The figure shows three views and two pictorial views of one solid part (mm, origin at its lowest corner). Answer the questions. A direction names the side the tool comes from. Round coordinates to 2 decimals unless told otherwise and drop trailing zeros. Loops run counter-clockwise (first coordinate to the right, second up) from the corner with the lowest first, then second, coordinate; pieces in that order, holes last. Notation, with made-up numbers: (-2, 54) -> (43, 54) arc R22 ccw to (43, 64) -> close; hole circle Ø2 at (22, 24.5). An arc over 180 degrees is marked (long way). Use a Markdown table: item, result. Add a question column.
Q1. For a pull along Y with two mould halves and no side action, classify the marked faces 3, 4 and 5 as released by +Y, released by -Y, zero draft, split by the parting line, or undercut.
Q2. Which of the six approach directions +Z, -Z, +X, -X, +Y, -Y give full straight-line access (tool end or side, diameter ignored) to the marked faces 1 and 2?
Q3. Section D-D on z = 14 is taken. Give the vertices of the cut face in (x, y).
Q4. Section C-C on z = 8 is taken. Give the vertices of the cut face in (x, y), then the cut area to 3 significant figures.
Q5. Section A-A on y = 10.5 is taken. Give the vertices of the cut face in (x, z).
Q6. Given pin 1 Ø6.5 at (y, z) = (10.5, 8) entering from -X; pin 2 Ø2 at (y, z) = (8, 6.5) entering from +X, each flat-ended and moving along its own axis, determine where each tip first touches the part or whether it passes through.
Q7. Section B-B on x = 9 is taken. Give the vertices of the cut face in (y, z), then the cut area to 3 significant figures.
Q8. Consider line 1 (X direction, y = 9.75, z = 3); line 2 (Y direction, x = 0.95, z = 8); line 3 (Y direction, x = 9.75, z = 13.5). Determine where each line is inside the solid, lowest interval first.
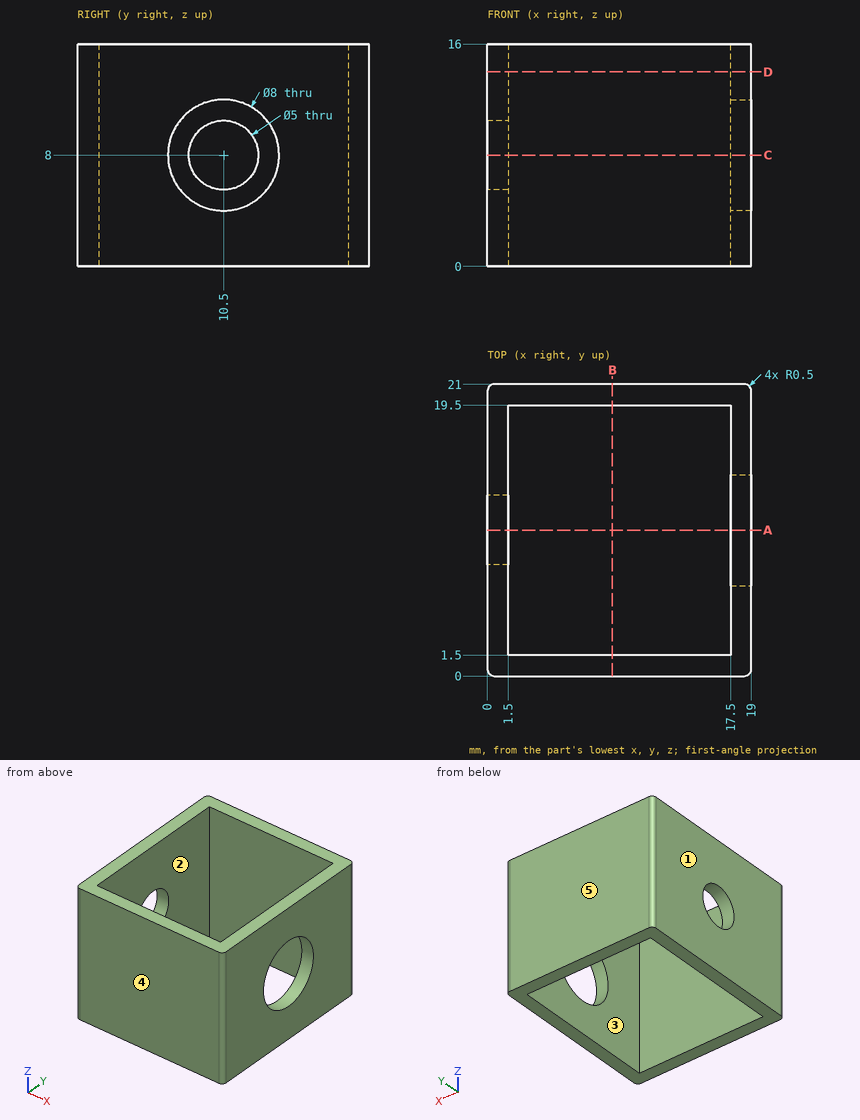
Checked values:
| question | item | result |
|---|---|---|
| 1 | face 3 | undercut |
| 1 | face 4 | released by -Y |
| 1 | face 5 | released by +Y |
| 2 | face 1 | +Z, -Z, -X, +Y, -Y |
| 2 | face 2 | +Z, -Z |
| 3 | outline | (0, 0.5) arc R0.5 ccw to (0.5, 0) -> (18.5, 0) arc R0.5 ccw to (19, 0.5) -> (19, 20.5) arc R0.5 ccw to (18.5, 21) -> (0.5, 21) arc R0.5 ccw to (0, 20.5) -> close; hole (1.5, 1.5) -> (17.5, 1.5) -> (17.5, 19.5) -> (1.5, 19.5) -> close |
| 4 | outline | (0, 0.5) arc R0.5 ccw to (0.5, 0) -> (18.5, 0) arc R0.5 ccw to (19, 0.5) -> (19, 6.5) -> (17.5, 6.5) -> (17.5, 1.5) -> (1.5, 1.5) -> (1.5, 8) -> (0, 8) -> close; (0, 13) -> (1.5, 13) -> (1.5, 19.5) -> (17.5, 19.5) -> (17.5, 14.5) -> (19, 14.5) -> (19, 20.5) arc R0.5 ccw to (18.5, 21) -> (0.5, 21) arc R0.5 ccw to (0, 20.5) -> close |
| 4 | area | 91.3 mm2 |
| 5 | outline | (0, 0) -> (1.5, 0) -> (1.5, 5.5) -> (0, 5.5) -> close; (0, 10.5) -> (1.5, 10.5) -> (1.5, 16) -> (0, 16) -> close; (17.5, 0) -> (19, 0) -> (19, 4) -> (17.5, 4) -> close; (17.5, 12) -> (19, 12) -> (19, 16) -> (17.5, 16) -> close |
| 6 | pin 1 | stops at x = 0 |
| 6 | pin 2 | stops at x = 1.5 |
| 7 | outline | (0, 0) -> (1.5, 0) -> (1.5, 16) -> (0, 16) -> close; (19.5, 0) -> (21, 0) -> (21, 16) -> (19.5, 16) -> close |
| 7 | area | 48.0 mm2 |
| 8 | line 1 | x = 0 to 1.5, 17.5 to 19 |
| 8 | line 2 | y = 0 to 8, 13 to 21 |
| 8 | line 3 | y = 0 to 1.5, 19.5 to 21 |
